```python
from build123d import *

# Parameters (mm, degrees)
ESQUISSE5_W                  = 4.75
ESQUISSE5_H                  = 4.75
BOSS_EXTRU_3_DEPTH           = 4
BOSS_EXTRU_4_DEPTH           = 4
ESQUISSE10_R                 = 4.375
ENL_V_MAT_EXTRU_2_DEPTH      = 50
ENL_V_MAT_EXTRU_3_DEPTH      = 50
ENL_V_MAT_EXTRU_3_DEPTH_BACK = 50
ESQUISSE11_R                 = 4.375


with BuildPart() as part:
    # Esquisse1 → Révolution1 (revolve)
    with BuildSketch(Plane(origin=(0, 0, 0), x_dir=(1, 0, 0), z_dir=(0, 1, 0))):
        Polygon((0, 0), (0, 4.75), (142, 4.75), (142, 0), (133.5, 0), (133.5, -26.75), (17, -26.75), (17, 0), align=None)
    revolve(axis=Axis((0, 0, -4.75), (1, 0, 0)))

    # Esquisse5 → Boss.-Extru.3 (add)
    with BuildSketch(Plane(origin=(142, 0, 0), x_dir=(0, 0, -1), z_dir=(1, 0, 0))):
        with Locations((4.75, 0)):
            Rectangle(ESQUISSE5_W, ESQUISSE5_H)
    extrude(amount=BOSS_EXTRU_3_DEPTH)

    # Esquisse6 → Boss.-Extru.4 (add)
    with BuildSketch(Plane.ZY):
        Polygon((-4.75, 2.375), (-7.125, 2.375), (-7.125, -2.375), (-2.375, -2.375), (-2.375, 2.375), align=None)
    extrude(amount=BOSS_EXTRU_4_DEPTH)

    # Esquisse10 → Enlèv. mat.-Extru.2 (cut)
    with BuildSketch(Plane.XY):
        Polygon((63.31, 0), (67.155, -6.659735355), (74.845, -6.659735355), (78.69, 0), (74.845, 6.659735355), (67.155, 6.659735355), align=None)
        with Locations((71, 0)):
            Circle(ESQUISSE10_R, mode=Mode.SUBTRACT)
    extrude(amount=-ENL_V_MAT_EXTRU_2_DEPTH, mode=Mode.SUBTRACT)

    # Esquisse11 → Enlèv. mat.-Extru.3 (cut, two sides: drawn at the far end of the back side and taken through both)
    with BuildSketch(Plane.XY.offset(-ENL_V_MAT_EXTRU_3_DEPTH_BACK)):
        with Locations((71, 0)):
            Circle(ESQUISSE11_R)
    extrude(amount=ENL_V_MAT_EXTRU_3_DEPTH + ENL_V_MAT_EXTRU_3_DEPTH_BACK, mode=Mode.SUBTRACT)


solid = part.part
```
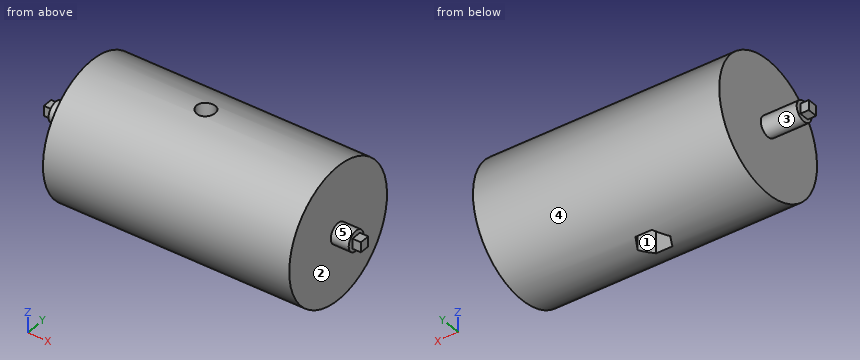
CAD build for the part. Positions are in the model's coordinates, mm. Face numbers are marked on the shaded views. A direction names the side the tool comes from. Round coordinates to 2 decimals unless told otherwise and drop trailing zeros. Write each loop counter-clockwise with the first axis right and the second up, starting at its lowest first coordinate (ties: lowest second). Pieces come first, ordered by that corner, then holes. Notation, with made-up numbers: (-6.75, 66.5) -> (14.25, 66.5) arc R10 cw to (14.25, 84.5) -> close; hole circle Ø1 at (16.25, 67.5). An arc over 180 degrees is marked (long way). Answer in a Markdown table with one row per item. Add a question column.
Item 1: Drop flat-ended pins along their axis: pin 1 Ø1 at (x, y) = (35.5, -23) entering from -Z; pin 2 Ø4 at (x, y) = (69, -2) entering from -Z; pin 3 Ø8.5 at (x, z) = (71.5, -25.5) entering from -Y; pin 4 Ø10.5 at (y, z) = (-2.5, -5.5) entering from +X. Give the stop position or say it passes through.
Item 2: Which spindle directions (+Z, -Z, +X, -X, +Y, -Y) get a long thin tool onto all of the face, cutting with end or side? Do the marked faces 4 and 5. Say none if no direction does.
Item 3: Mould opens along Y. For the marked faces 1, 2 and 3 say: pulls with the +Y half, pulls with the -Y half, needs draft (parallel to the pull), parting line crosses it, or undercut.
Item 4: Saw through at B-B, the plane x = 71. Write the cut outline in (y, z) (3 decimals), then the cut area to 3 significant figures.
Item 5: Saw through at A-A, the plane z = -4.75. Write the cut outline in (x, y) (3 decimals), then the cut area to 3 significant figures.
Item 6: Saw through at D-D, the plane z = -22. Write the cut outline in (x, y) (3 decimals).
Item 7: Saw through at C-C, the plane x = 114. Write the cut outline in (y, z).
Item 8: Drill centre lines: line 1 (X direction, y = 0, z = 11.75) (3 decimals); line 2 (X direction, y = 0.5, z = 18); line 3 (X direction, y = -20, z = 17). Where is each one in solid material? Low to high. Write a range as from..to.
Findings below:
| question | item | result |
|---|---|---|
| 1 | pin 1 | stops at z = -26.8 |
| 1 | pin 2 | stops at z = 0 |
| 1 | pin 3 | stops at y = -26.83 |
| 1 | pin 4 | stops at x = 146 |
| 2 | face 4 | +X, -X |
| 2 | face 5 | +X |
| 3 | face 1 | undercut |
| 3 | face 2 | needs draft |
| 3 | face 3 | parting line crosses it |
| 4 | outline | (-6.66, -35.538) -> (-6.66, 0) -> (-4.375, 0) -> (-4.375, 26.445) arc R31.5 ccw to start; (4.375, 0) -> (6.66, 0) -> (6.66, -35.538) arc R31.5 ccw to (4.375, 26.445) -> close |
| 4 | area | 2,400 mm^2 |
| 5 | outline | (-4, -2.375) -> (0, -2.375) -> (0, -4.75) -> (17, -4.75) -> (17, -31.5) -> (133.5, -31.5) -> (133.5, -4.75) -> (142, -4.75) -> (142, -2.375) -> (146, -2.375) -> (146, 2.375) -> (142, 2.375) -> (142, 4.75) -> (133.5, 4.75) -> (133.5, 31.5) -> (17, 31.5) -> (17, 4.75) -> (0, 4.75) -> (0, 2.375) -> (-4, 2.375) -> close; hole (63.31, 0) -> (67.155, -6.66) -> (74.845, -6.66) -> (78.69, 0) -> (74.845, 6.66) -> (67.155, 6.66) -> close |
| 5 | area | 7,470 mm^2 |
| 6 | outline | (17, -26.357) -> (133.5, -26.357) -> (133.5, 26.357) -> (17, 26.357) -> close; hole (63.31, 0) -> (67.155, -6.66) -> (74.845, -6.66) -> (78.69, 0) -> (74.845, 6.66) -> (67.155, 6.66) -> close |
| 7 | outline | circle Ø63 at (0, -4.75) |
| 8 | line 1 | x = 17..66.625, 75.375..133.5 |
| 8 | line 2 | x = 17..66.65, 75.35..133.5 |
| 8 | line 3 | x = 17..133.5 |
